Build history of the part. All positions in model axes, mm. A direction names the side the tool comes from. Round coordinates to 2 decimals unless told otherwise and drop trailing zeros. Write each loop counter-clockwise with the first axis right and the second up, starting at its lowest first coordinate (ties: lowest second). Pieces come first, ordered by that corner, then holes. Notation, with made-up numbers: (36, 82) -> (69, 82) arc R30 cw to (69, 118) -> close; hole circle Ø2 at (-19.5, 58). An arc over 180 degrees is marked (long way). Answer in a Markdown table with one row per item.
```python
from build123d import *

# Parameters (mm, degrees)
SKETCH_1_W             = 35
SKETCH_1_H             = 60
SKETCH_1_R             = 13.5
EXTRUDE_1_DEPTH        = 10
SKETCH_3_R             = 13.5
SKETCH_3_R_2           = 11.5
EXTRUDE_2_DEPTH        = 2
HOLE_WIZARD_M4_2_D     = 3.3
HOLE_WIZARD_M4_2_DEPTH = 11.5
HOLE_WIZARD_M4_2_TIP   = 0.991420021
HOLE_WIZARD_M4_3_D     = 3.3
HOLE_WIZARD_M4_3_DEPTH = 11.5
HOLE_WIZARD_M4_3_TIP   = 0.991420021


with BuildPart() as part:
    # 스케치1 → 보스-돌출1 (new body)
    with BuildSketch(Plane(origin=(0, 0, 0), x_dir=(1, 0, 0), z_dir=(0, 1, 0))):
        Rectangle(SKETCH_1_W, SKETCH_1_H)
        Circle(SKETCH_1_R, mode=Mode.SUBTRACT)
    extrude(amount=EXTRUDE_1_DEPTH)

    # 스케치3 → 보스-돌출2 (add)
    with BuildSketch(Plane(origin=(0, 10, 0), x_dir=(1, 0, 0), z_dir=(0, 1, 0))):
        Circle(SKETCH_3_R)
        Circle(SKETCH_3_R_2, mode=Mode.SUBTRACT)
    extrude(amount=-EXTRUDE_2_DEPTH)

    # M4 나사 구멍2
    with Locations(Plane.XY.offset(30)):
        with Locations((-8, 5), (0, 5), (8, 5)):
            Hole(HOLE_WIZARD_M4_2_D / 2, depth=HOLE_WIZARD_M4_2_DEPTH)
            with Locations((0, 0, -(HOLE_WIZARD_M4_2_DEPTH + HOLE_WIZARD_M4_2_TIP / 2))):  # 118° drill point
                Cone(0, HOLE_WIZARD_M4_2_D / 2, HOLE_WIZARD_M4_2_TIP, mode=Mode.SUBTRACT)

    # M4 나사 구멍3
    with Locations(Plane(origin=(0, 0, -30), x_dir=(-1, 0, 0), z_dir=(0, 0, -1))):
        with Locations((-8, 5), (0, 5), (8, 5)):
            Hole(HOLE_WIZARD_M4_3_D / 2, depth=HOLE_WIZARD_M4_3_DEPTH)
            with Locations((0, 0, -(HOLE_WIZARD_M4_3_DEPTH + HOLE_WIZARD_M4_3_TIP / 2))):  # 118° drill point
                Cone(0, HOLE_WIZARD_M4_3_D / 2, HOLE_WIZARD_M4_3_TIP, mode=Mode.SUBTRACT)


solid = part.part
```
Q1. Wall check: line 1 (X direction, y = 5, z = 25.5); line 2 (Z direction, x = 0, y = 9.1); line 3 (Y direction, x = 8, z = -22.25). Give the ranges that are in metal, low to high. Write a range as [from, to].
A:
| item | result |
|---|---|
| line 1 | [-17.5, -9.65], [-6.35, -1.65], [1.65, 6.35], [9.65, 17.5] |
| line 2 | [-30, -11.5], [11.5, 30] |
| line 3 | [0, 3.35], [6.65, 10] |
Q2. Which spindle directions (+Z, -Z, +X, -X, +Y, -Y) get a long thin tool onto all of the face, cutting with end or side? Do faces 5 (the flat face through (0, 3, 30)), 6 (the cylindrical face through (-8.4, 3.4, -24.2)), 7 (the flat face through (0, 3, -30)), 8 (the flat face through (10, 8, -6)), 9 (the cylindrical face through (8.4, 3.4, 24.2)). Say none if no direction does.
A:
| item | result |
|---|---|
| face 5 | +Z, +X, -X, +Y, -Y |
| face 6 | -Z |
| face 7 | -Z, +X, -X, +Y, -Y |
| face 8 | -Y |
| face 9 | +Z |
Q3. Two-plate mould, pull along X, no slides. Class faces 1 (the flat face through (-12, 10, 0)), 2 (the flat face through (17.5, 5, 0)), 3 (the flat face through (-17.5, 5, 0)), 4 (the conical face through (8.3, 5.1, 17.7)): released by +X, released by -X, zero draft, split by the parting line, or undercut.
A:
| item | result |
|---|---|
| face 1 | zero draft |
| face 2 | released by +X |
| face 3 | released by -X |
| face 4 | undercut |
Q4. Saw through at C-C on z = 20. Write the cut outline in (x, y), plus the area to 3 significant figures.
A:
| item | result |
|---|---|
| outline | (-17.5, 0) -> (17.5, 0) -> (17.5, 10) -> (-17.5, 10) -> close; hole circle Ø3.3 at (-8, 5); hole circle Ø3.3 at (0, 5); hole circle Ø3.3 at (8, 5) |
| area | 324 mm² |
Q5. Saw through at B-B on x = -4. Write the cut outline in (y, z).
A:
| item | result |
|---|---|
| outline | (0, -30) -> (10, -30) -> (10, -10.78) -> (8, -10.78) -> (8, -12.89) -> (0, -12.89) -> close; (0, 12.89) -> (8, 12.89) -> (8, 10.78) -> (10, 10.78) -> (10, 30) -> (0, 30) -> close |
Q6. Saw through at A-A on z = 0. Write the cut outline in (x, y), plus the area to 3 significant figures.
A:
| item | result |
|---|---|
| outline | (-17.5, 0) -> (-13.5, 0) -> (-13.5, 8) -> (-11.5, 8) -> (-11.5, 10) -> (-17.5, 10) -> close; (11.5, 8) -> (13.5, 8) -> (13.5, 0) -> (17.5, 0) -> (17.5, 10) -> (11.5, 10) -> close |
| area | 88.0 mm² |
Q7. Drop flat-ended pins along their axis: P1, Ø2, axis at x = 8, y = 5, coming from the -Z side; P2, Ø2.5, axis at x = -8, y = 5, coming from the -Z side; P3, Ø2, axis at x = -8, y = 5, coming from the +Z side. Give the stop position or say it passes through.
A:
| item | result |
|---|---|
| P1 | z = -18.11 |
| P2 | z = -18.26 |
| P3 | z = 18.11 |
Q8. Saw through at D-D on y = 2.5. Write the cut outline in (x, z), plus the area to 3 significant figures.
A:
| item | result |
|---|---|
| outline | (-17.5, -30) -> (17.5, -30) -> (17.5, 30) -> (-17.5, 30) -> close; hole circle Ø27 at (0, 0) |
| area | 1,530 mm² |
